CAD build for the part. Positions are in the model's coordinates, mm. A direction names the side the tool comes from. Give positions to 0.01 mm unless a question says otherwise; leave off trailing zeros. Loops run counter-clockwise (first coordinate to the right, second up) from the corner with the lowest first, then second, coordinate; pieces in that order, holes last.
```python
from build123d import *

# Parameters (mm, degrees)
SKETCH1_W          = 8.5
SKETCH1_H          = 134
SKETCH2_W          = 3.25
SKETCH2_H          = 3.25
CUT_EXTRUDE1_DEPTH = 30
CHAMFER1_SIZE      = 0.5
SKETCH4_OUTSIDE_W  = 46.228
SKETCH4_OUTSIDE_H  = 46.228
SKETCH4_OUTSIDE_R  = 8
CUT_EXTRUDE3_DEPTH = 30
SKETCH3_W          = 3.25
SKETCH3_H          = 3.25
CUT_EXTRUDE2_DEPTH = 25


with BuildPart() as part:
    # Sketch1 → Revolve1 (revolve)
    with BuildSketch(Plane.XY, mode=Mode.PRIVATE) as revolve1_sk:
        with Locations((4.25, 67)):
            Rectangle(SKETCH1_W, SKETCH1_H)
    revolve(revolve1_sk.sketch.rotate(Axis((0, 134, 0), (0, -1, 0)), 90), axis=Axis((0, 134, 0), (0, -1, 0)))

    # Sketch2 → Cut-Extrude1 (cut)
    with BuildSketch(Plane.XZ):
        with Locations((0, 8.5)):
            Rectangle(SKETCH2_W, SKETCH2_H)
    extrude(amount=-CUT_EXTRUDE1_DEPTH, mode=Mode.SUBTRACT)

    # Chamfer1
    chamfer1_edges = [part.edges().sort_by_distance(p)[0] for p in [
        (1.625, 0, 7.609111649),
        (0, 0, 6.875),
        (0, 0, -8.5),
        (0, 134, -8.5),
        (-1.625, 0, 7.609111649),
    ]]
    chamfer(chamfer1_edges, length=CHAMFER1_SIZE)

    # Sketch4 outside → Cut-Extrude3 (cut)
    with BuildSketch(Plane(origin=(0, 134, 0), x_dir=(1, 0, 0), z_dir=(0, 1, 0))):
        Rectangle(SKETCH4_OUTSIDE_W, SKETCH4_OUTSIDE_H)
        with Locations(Location((0, 0, 0), (0, 0, 180))):
            Circle(SKETCH4_OUTSIDE_R, mode=Mode.SUBTRACT)
    extrude(amount=-CUT_EXTRUDE3_DEPTH, mode=Mode.SUBTRACT)

    # Sketch3 → Cut-Extrude2 (cut)
    with BuildSketch(Plane(origin=(0, 134, 0), x_dir=(1, 0, 0), z_dir=(0, 1, 0))):
        with Locations((0, 8)):
            Rectangle(SKETCH3_W, SKETCH3_H)
    extrude(amount=-CUT_EXTRUDE2_DEPTH, mode=Mode.SUBTRACT)


solid = part.part
```
1. Saw through at A-A, the plane x = 0. List the corners of the cut face in (y, z) (3 decimals), and give its area (3 significant figures).
Responses:
outline: (0, -8) - (0.5, -8.5) - (104, -8.5) - (104, -8) - (109, -8) - (109, -6.375) - (134, -6.375) - (134, 8) - (104, 8) - (104, 8.5) - (30, 8.5) - (30, 6.875) - (0.5, 6.875) - (0, 6.375) - close
area: 2,160 mm2
2. Tool access for faces 1 (the face through (0, 134, 0)), 2 (the face through (0, 122, -6.375)): list every direction of +Z, -Z, +X, -X, +Y, -Y with a clear straight run to the whole face (end or side of a thin tool).
Responses:
face 1: +Z, -Z, +X, -X, +Y
face 2: -Z, +Y
3. Drop flat-ended pins along their axis: pin 1 (8 mm diameter, centred on x = -1, y = 110.5, fed in from -Z); pin 2 (0.8 mm diameter, centred on x = -0.5, z = -7, fed in from +Y); pin 3 (1 mm diameter, centred on y = 117.5, z = -5.5, fed in from -X) (3 decimals). Give the stop position or say it passes through.
Responses:
pin 1: stops at z = -8
pin 2: stops at y = 109
pin 3: stops at x = -6.245
4. Pull direction X, two halves, no side cores. Call faces 3 (the face through (0, 0, 0)), 4 (the face through (-3.69, 119.21, -7.1)), 5 (the face through (0, 15, 6.875)): released by +X, released by -X, zero draft, split by the parting line, or undercut.
Responses:
face 3: zero draft
face 4: split by the parting line
face 5: undercut
5. Saw through at B-B, the plane y = 85.5. List the corners of the cut face in (x, z), and give its area (3 significant figures).
Responses:
outline: circle Ø17 at (0, 0)
area: 227 mm2
6. Probe line 1 along Y through (x, z) = (-1, -6.5); line 2 along Y through (x, z) = (3.75, -7.25); line 3 along Z through (x, y) = (-1.25, 49). List the from-to ranges inside material, lowest first.
Responses:
line 1: y = 0 to 109
line 2: y = 0.16 to 104
line 3: z = -8.41 to 8.41
